Read the model definition and answer for the solid it produces. Units are mm, in the model's axes. Coordinates: 2 decimals unless noted, no trailing zeros. Write each loop counter-clockwise with the first axis right and the second up, starting at its lowest first coordinate (ties: lowest second). Pieces come first, ordered by that corner, then holes.
(1) The mould has two halves that part along X. Classify faces 1 (the cylindrical face through (11.46, 51.57, 6.27)), 2 (the flat face through (25.4, 28, 6)), 3 (the conical face through (12.971, 69.482, 0.135)), 4 (the flat face through (13, 35, 0)): +X half, -X half, draft (parallel to the pull), parting line (faces both ways), or undercut.
(2) Section A-A on x = 12.7 is taken. State how many separate pieces and enclosed holes the cut face has, then the cut area to 3 significant figures.
(3) Section B-B on z = 7.75 is taken. Write down the section's boundary in (x, y) (3 decimals), then the cut area to 3 significant figures.
(4) Given pin 1 (10 mm diameter, centred on x = 15, y = 17, fed in from -Z); pin 2 (4 mm diameter, centred on y = 59.5, z = 11, fed in from -X); pin 3 (2 mm diameter, centred on x = 19.5, z = 3.5, fed in from +Y); pin 4 (1 mm diameter, centred on x = 4.5, z = 1.5, fed in from +Y), each flat-ended and moving along its own axis, determine where each tip first touches the part or whether it passes through.
(5) Find the intervals of material crossed by probe 1 along Y at (x, z) = (12.7, 4.75) (3 decimals); probe 2 along Y at (x, z) = (10.75, 0.5); probe 3 along X at (y, z) = (56, 4.75), in increasing order.
from build123d import *

# Parameters (mm, degrees)
SKETCH1_R           = 5.715
SKETCH1_R_2         = 3.175
BOSS_EXTRUDE1_DEPTH = 12.7
CHAMFER1_SIZE       = 0.5


with BuildPart() as part:
    # Sketch1 → Boss-Extrude1 (new body)
    with BuildSketch(Plane.XY):
        with BuildLine():
            Line((0, 0), (25.4, 0))
            Line((25.4, 0), (25.4, 40.64))
            Line((25.4, 40.64), (25.4, 57.15))
            ThreePointArc((25.4, 57.15), (12.7, 69.85), (0, 57.15))
            Line((0, 57.15), (0, 40.64))
            Line((0, 40.64), (0, 0))
        make_face()
        with Locations((12.7, 57.15)):
            Circle(SKETCH1_R, mode=Mode.SUBTRACT)
        with Locations((12.7, 27.305)):
            Circle(SKETCH1_R_2, mode=Mode.SUBTRACT)
        with Locations((12.7, 12.065)):
            Circle(SKETCH1_R_2, mode=Mode.SUBTRACT)
    extrude(amount=BOSS_EXTRUDE1_DEPTH)

    # Chamfer1
    chamfer1_edges = [part.edges().sort_by_distance(p)[0] for p in [
        (25.4, 28.575, 12.7),
        (9.525, 27.305, 0),
        (9.525, 27.305, 12.7),
        (12.7, 69.85, 12.7),
        (6.985, 57.15, 0),
        (6.985, 57.15, 12.7),
        (9.525, 12.065, 0),
        (9.525, 12.065, 12.7),
        (0, 28.575, 12.7),
        (0, 28.575, 0),
        (12.7, 69.85, 0),
        (25.4, 28.575, 0),
        (12.7, 0, 0),
        (12.7, 0, 12.7),
    ]]
    chamfer(chamfer1_edges, length=CHAMFER1_SIZE)


solid = part.part
Response:
1. face 1: undercut
1. face 2: +X half
1. face 3: parting line
1. face 4: draft
2. separate pieces: 4
2. enclosed holes: 0
2. area: 579 mm2
3. outline: (0, 0) - (25.4, 0) - (25.4, 57.15) arc R12.7 ccw to (0, 57.15) - close; hole circle Ø11.43 at (12.7, 57.15); hole circle Ø6.35 at (12.7, 12.065); hole circle Ø6.35 at (12.7, 27.305)
3. area: 1,540 mm2
4. pin 1: stops at z = 0
4. pin 2: stops at x = 0
4. pin 3: stops at y = 68.45
4. pin 4: stops at y = 67.25
5. probe 1: y = 0 to 8.89, 15.24 to 24.13, 30.48 to 51.435, 62.865 to 69.85
5. probe 2: y = 0 to 9.56, 14.57 to 24.8, 29.81 to 51.78, 62.52 to 69.7
5. probe 3: x = 0 to 7.1, 18.3 to 25.4
